from build123d import *

# Parameters (mm, degrees)
F3_D     = 12.7
F4_W     = 60
F4_H     = 90
F4_R     = 6.35
F5_DEPTH = 10
F6_R     = 1
F7_DEPTH = 10
F8_R     = 1
F9_DEPTH = 10
F10_R    = 0.5


with BuildPart() as f1:
    # F0 (on Front) → F1 (revolve)
    with BuildSketch(Plane.XZ):
        Polygon((0, 30), (0, 0), (92.5, 0), (42.4, 30), align=None)
    revolve(axis=Axis((0, 0, 15), (0, 0, 1)))

    # F3 (through all)
    with Locations(Plane.XY.offset(30)):
        with Locations((0, 0)):
            Hole(F3_D / 2)

    # F4 (on face) → F5 (cut)
    with BuildSketch(Plane(origin=(0, 0, 0), x_dir=(1, 0, 0), z_dir=(0, 0, -1))):
        with Locations((0.233456, -0.599967)):
            Rectangle(F4_W, F4_H)
        Circle(F4_R, mode=Mode.SUBTRACT)
    extrude(amount=-F5_DEPTH, mode=Mode.SUBTRACT)

    # F6 (on face) → F7 (cut)
    with BuildSketch(Plane(origin=(0, 0, 0), x_dir=(1, 0, 0), z_dir=(0, 0, -1))):
        with Locations((-44.5, 0)):
            Circle(F6_R)
        with Locations((44.5, 0)):
            Circle(F6_R)
    extrude(amount=-F7_DEPTH, mode=Mode.SUBTRACT)

    # F8 (on face) → F9 (cut)
    with BuildSketch(Plane.XY.offset(30)):
        with Locations((-25.4, 0)):
            Circle(F8_R)
        with Locations((25.4, 0)):
            Circle(F8_R)
    extrude(amount=-F9_DEPTH, mode=Mode.SUBTRACT)

    # F10
    f10_edges = [f1.edges().sort_by_distance(p)[0] for p in [
        (-92.5, 0, 0),
        (-42.4, 0, 30),
    ]]
    fillet(f10_edges, radius=F10_R)


solid = f1.part
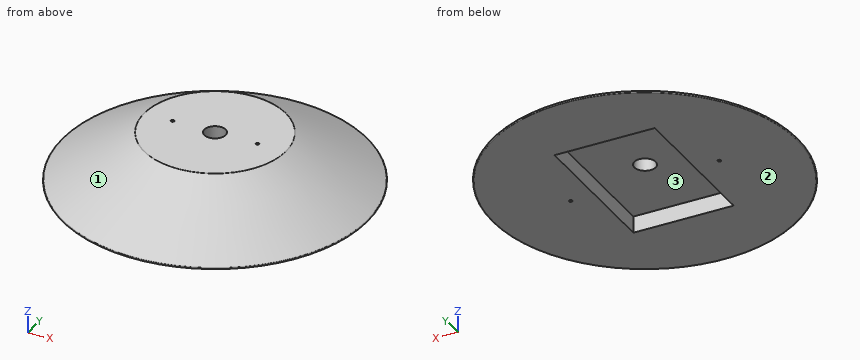
The listing builds one solid part. Answer for the finished solid, in the listing's coordinates (mm). Face numbers are marked on the shaded views. Coordinates: 2 decimals unless noted, no trailing zeros. Loops run counter-clockwise (first coordinate to the right, second up) from the corner with the lowest first, then second, coordinate; pieces in that order, holes last. Notation, with made-up numbers: (-11.5, 47.25) -> (12.5, 47.25) arc R5 cw to (12.5, 51.25) -> close; hole circle Ø4 at (63, -19.5). An arc over 180 degrees is marked (long way). Answer in a Markdown table with one row per item. Add a question column.
1. Determine the mould class of the marked faces 1, 2 and 3 for opening direction Y: +Y half, -Y half, draft (parallel to the pull), parting line (faces both ways), or undercut.
2. Flat-ended cylindrical pins translate along their axes: P1, Ø10, axis at y = -17, z = 6.5, coming from the +X side; P2, Ø0.6, axis at x = -26, y = 0, coming from the +Z side; P3, Ø2.5, axis at x = -25.4, y = 0, coming from the +Z side; P4, Ø8, axis at x = 46.5, y = 40.5, coming from the +Z side. Find the tip coordinate at first contact, or state that the pin passes through.
3. Consider line 1 (Y direction, x = -44.5, z = 2); line 2 (Z direction, x = 11, y = 3); line 3 (Y direction, x = 28, z = 5). Determine where each line is inside the solid, lowest interval first. Write a range as [from, to].
4. The part is cut by section B-B, the plane z = 16. Write down the section's boundary in (x, y).
5. The part is cut by section A-A, the plane x = 0. Write down the section's boundary in (y, z), then the cut area to 3 significant figures.
6. The part is cut by section C-C, the plane z = 27.5. Write down the section's boundary in (x, y) (3 decimals), then the cut area to 3 significant figures.
Answer below:
| question | item | result |
|---|---|---|
| 1 | face 1 | parting line |
| 1 | face 2 | draft |
| 1 | face 3 | undercut |
| 2 | P1 | x = 88.43 |
| 2 | P2 | z = 20 |
| 2 | P3 | z = 30 |
| 2 | P4 | z = 20.86 |
| 3 | line 1 | [-77.26, -1], [1, 77.26] |
| 3 | line 2 | [10, 30] |
| 3 | line 3 | [-79.36, -44.4], [45.6, 79.36] |
| 4 | outline | circle Ø131.56 at (0, 0); hole circle Ø12.7 at (0, 0) |
| 5 | outline | (-90.95, 0.93) arc R0.5 ccw to (-90.69, 0) -> (-44.4, 0) -> (-44.4, 10) -> (-6.35, 10) -> (-6.35, 30) -> (-42.26, 30) arc R0.5 ccw to (-42.52, 29.93) -> close; (6.35, 10) -> (45.6, 10) -> (45.6, 0) -> (90.69, 0) arc R0.5 ccw to (90.95, 0.93) -> (42.52, 29.93) arc R0.5 ccw to (42.26, 30) -> (6.35, 30) -> close |
| 5 | area | 2,890 mm2 |
| 6 | outline | circle Ø93.15 at (0, 0); hole circle Ø2 at (-25.4, 0); hole circle Ø12.7 at (0, 0); hole circle Ø2 at (25.4, 0) |
| 6 | area | 6,680 mm2 |
